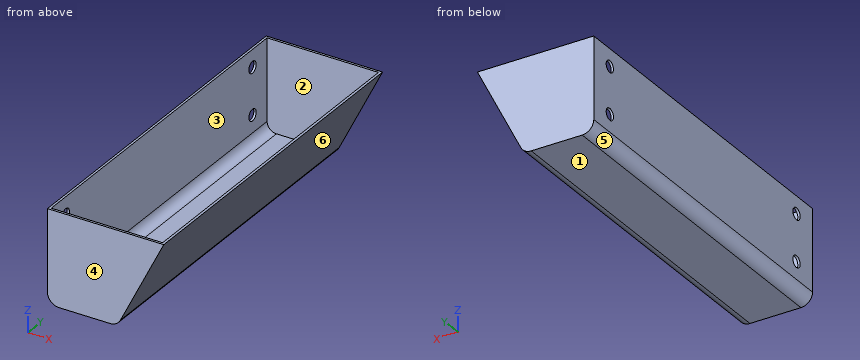
from build123d import *

# Parameters (mm, degrees)
BOSS_EXTRUDE1_DEPTH = 75
SHELL1_T            = -1
CUT_EXTRUDE1_REACH  = 100.112
SKETCH3_R           = 2.5


with BuildPart() as part:
    # Sketch2 → Boss-Extrude1 (new, symmetric)
    with BuildSketch(Plane(origin=(0, 0, 0), x_dir=(-1, 0, 0), z_dir=(0, 1, 0))):
        with BuildLine():
            Line((0, 40), (0, 5))
            ThreePointArc((0, 5), (-1.464466094, 1.464466094), (-5, 0))
            Line((-5, 0), (-26.909830056, 0))
            ThreePointArc((-26.909830056, 0), (-29.538485617, 0.746745958), (-31.381966011, 2.763932023))
            Line((-31.381966011, 2.763932023), (-50, 40))
            Line((-50, 40), (0, 40))
        make_face()
    extrude(amount=BOSS_EXTRUDE1_DEPTH, both=True)

    # Shell1
    shell1_openings = [part.faces().sort_by_distance(p)[0] for p in [
        (25, 0, 40),
    ]]
    offset(amount=SHELL1_T, openings=shell1_openings, kind=Kind.INTERSECTION)

    # Sketch3 → Cut-Extrude1 (cut, up to next)
    with BuildSketch(Plane.YZ.offset(1), mode=Mode.PRIVATE) as cut_extrude1_sk1:
        with Locations(Location((-64, 32.5, 0), (0, 0, 270))):
            Circle(SKETCH3_R)
    cut_extrude1_tool1 = extrude(cut_extrude1_sk1.sketch, amount=-CUT_EXTRUDE1_REACH, mode=Mode.PRIVATE) & part.part
    # Sketch3 → Cut-Extrude1 (cut, up to next)
    with BuildSketch(Plane.YZ.offset(1), mode=Mode.PRIVATE) as cut_extrude1_sk2:
        with Locations(Location((-64, 12.5, 0), (0, 0, 270))):
            Circle(SKETCH3_R)
    cut_extrude1_tool2 = extrude(cut_extrude1_sk2.sketch, amount=-CUT_EXTRUDE1_REACH, mode=Mode.PRIVATE) & part.part
    # Sketch3 → Cut-Extrude1 (cut, up to next)
    with BuildSketch(Plane.YZ.offset(1), mode=Mode.PRIVATE) as cut_extrude1_sk3:
        with Locations(Location((64, 12.5, 0), (0, 0, 270))):
            Circle(SKETCH3_R)
    cut_extrude1_tool3 = extrude(cut_extrude1_sk3.sketch, amount=-CUT_EXTRUDE1_REACH, mode=Mode.PRIVATE) & part.part
    # Sketch3 → Cut-Extrude1 (cut, up to next)
    with BuildSketch(Plane.YZ.offset(1), mode=Mode.PRIVATE) as cut_extrude1_sk4:
        with Locations(Location((64, 32.5, 0), (0, 0, 270))):
            Circle(SKETCH3_R)
    cut_extrude1_tool4 = extrude(cut_extrude1_sk4.sketch, amount=-CUT_EXTRUDE1_REACH, mode=Mode.PRIVATE) & part.part
    add(cut_extrude1_tool1.solids().sort_by_distance((1, -64, 32.5))[0], mode=Mode.SUBTRACT)
    add(cut_extrude1_tool2.solids().sort_by_distance((1, -64, 12.5))[0], mode=Mode.SUBTRACT)
    add(cut_extrude1_tool3.solids().sort_by_distance((1, 64, 12.5))[0], mode=Mode.SUBTRACT)
    add(cut_extrude1_tool4.solids().sort_by_distance((1, 64, 32.5))[0], mode=Mode.SUBTRACT)


solid = part.part
Work out the finished part from the listing and answer in its coordinate system (mm). Face numbers are marked on the shaded views. A direction names the side the tool comes from. Round coordinates to 2 decimals unless told otherwise and drop trailing zeros. Write each loop counter-clockwise with the first axis right and the second up, starting at its lowest first coordinate (ties: lowest second). Pieces come first, ordered by that corner, then holes. Notation, with made-up numbers: (-25.75, 88.5) - (-6.75, 88.5) arc R26 ccw to (-6.75, 102.5) - close; hole circle Ø8 at (-14.75, 16). An arc over 180 degrees is marked (long way). Answer in a Markdown table with one row per item. Add a question column.
1. A cutting plane is placed at B-B, the plane z = 32.5. Determine the outline of the cut face in (x, y), and give its area (3 significant figures).
2. A cutting plane is placed at C-C, the plane y = 10. Determine the outline of the cut face in (x, z), and give its area (3 significant figures).
3. For the marked faces 1 and 2, determine the directions among +Z, -Z, +X, -X, +Y, -Y from which every point of the face is accessible in a straight line to the end or side of a thin tool.
4. A cutting plane is placed at D-D, the plane x = 22.5. Determine the outline of the cut face in (y, z).
5. The mould has two halves that part along X. Classify the marked faces 3, 4, 5 and 6: +X half, -X half, draft (parallel to the pull), parting line (faces both ways), or undercut.
6. Find the intervals of material crossed by line 1 along Y through (x, z) = (0.75, 12.5); line 2 along Y through (x, z) = (25, 21); line 3 along Z through (x, y) = (24, -24.5), in increasing order. Write a range as from..to.
7. Given pin 1 (2 mm diameter, centred on y = -31, z = 11, fed in from +X); pin 2 (11 mm diameter, centred on x = 19.5, y = -11, fed in from +Z); pin 3 (8 mm diameter, centred on x = 39, y = 18, fed in from +Z), each flat-ended and moving along its own axis, determine where each tip first touches the part or whether it passes through.
8. A cutting plane is placed at A-A, the plane y = -64. Determine the outline of the cut face in (x, z).
Worked out:
| question | item | result |
|---|---|---|
| 1 | outline | (0, -75) - (46.25, -75) - (46.25, 75) - (0, 75) - (0, 66.5) - (1, 66.5) - (1, 74) - (45.13, 74) - (45.13, -74) - (1, -74) - (1, -66.5) - (0, -66.5) - close; (0, -61.5) - (1, -61.5) - (1, 61.5) - (0, 61.5) - close |
| 1 | area | 396 mm^2 |
| 2 | outline | (0, 5) arc R5 ccw to (5, 0) - (26.91, 0) arc R5 ccw to (31.38, 2.76) - (50, 40) - (48.88, 40) - (30.49, 3.21) arc R4 cw to (26.91, 1) - (5, 1) arc R4 cw to (1, 5) - (1, 40) - (0, 40) - close |
| 2 | area | 110 mm^2 |
| 3 | face 1 | -Z, +X, -X, +Y, -Y |
| 3 | face 2 | +Z |
| 4 | outline | (-75, 0) - (75, 0) - (75, 40) - (74, 40) - (74, 1) - (-74, 1) - (-74, 40) - (-75, 40) - close |
| 5 | face 3 | undercut |
| 5 | face 4 | draft |
| 5 | face 5 | -X half |
| 5 | face 6 | +X half |
| 6 | line 1 | -75..-66.5, -61.5..61.5, 66.5..75 |
| 6 | line 2 | -75..-74, 74..75 |
| 6 | line 3 | 0..1 |
| 7 | pin 1 | x = 36 |
| 7 | pin 2 | z = 1 |
| 7 | pin 3 | z = 28.24 |
| 8 | outline | (0, 5) arc R5 ccw to (5, 0) - (26.91, 0) arc R5 ccw to (31.38, 2.76) - (50, 40) - (48.88, 40) - (30.49, 3.21) arc R4 cw to (26.91, 1) - (5, 1) arc R4 cw to (1, 5) - (1, 10) - (0, 10) - close; (0, 15) - (1, 15) - (1, 30) - (0, 30) - close; (0, 35) - (1, 35) - (1, 40) - (0, 40) - close |
